```python
from build123d import *

# Parameters (mm, degrees)
PAD_DEPTH       = 5
CHAMFER_SIZE    = 3
SKETCH001_R     = 1.65
POCKET_DEPTH    = 5
FILLET_R        = 4
SKETCH002_R     = 1.7
POCKET001_DEPTH = 10.001
CHAMFER001_SIZE = 1.5


with BuildPart() as part:
    # Sketch → Pad (new body, symmetric)
    with BuildSketch(Plane.XY):
        Polygon((-27.5, 0), (0, 0), (0, 30), (-9, 30), (-9, 4), (-27.5, 4), align=None)
    extrude(amount=PAD_DEPTH, both=True)

    # Chamfer
    chamfer_edges = [part.edges().sort_by_distance(p)[0] for p in [
        (0, 0, 0),
    ]]
    chamfer(chamfer_edges, length=CHAMFER_SIZE)

    # Sketch001 (on Face7 of Chamfer) → Pocket (cut)
    with BuildSketch(Plane(origin=(0, 4, 0), x_dir=(-1, 0, 0), z_dir=(0, 1, 0))):
        with Locations((22.75, 0)):
            Circle(SKETCH001_R)
        with Locations((13.75, 0)):
            Circle(SKETCH001_R)
    extrude(amount=-POCKET_DEPTH, mode=Mode.SUBTRACT)

    # Fillet
    fillet_edges = [part.edges().sort_by_distance(p)[0] for p in [
        (-9, 30, 0),
        (0, 30, 0),
    ]]
    fillet(fillet_edges, radius=FILLET_R)

    # Sketch002 (on Face11 of Fillet) → Pocket001 (cut, through all)
    with BuildSketch(Plane.XY.offset(5)):
        with Locations((-4.5, 25)):
            Circle(SKETCH002_R)
    extrude(amount=-POCKET001_DEPTH, mode=Mode.SUBTRACT)

    # Chamfer001
    chamfer001_edges = [part.edges().sort_by_distance(p)[0] for p in [
        (-27.5, 4, 0),
    ]]
    chamfer(chamfer001_edges, length=CHAMFER001_SIZE)


solid = part.part
```
Geometry check sheet. Reference: the model listing, model coordinates, mm. A direction names the side the tool comes from. Give positions to 0.01 mm unless a question says otherwise; leave off trailing zeros. Order: outer loops, then holes, each group sorted by start corner. A loop starts at its lowest first (then second) coordinate and runs counter-clockwise, first axis right, second up.
1. Release check for a two-part mould opening along X. For faces 1 (the face through (-8, 12, -5)), 2 (the face through (-15.274, 2.028, -0.632)), 3 (the face through (-7.797, 28.859, 0.07)), 4 (the face through (-1, 2, 0)) record: pulls with the +X half, pulls with the -X half, needs draft (parallel to the pull), parting line crosses it, or undercut.
2. Section check B-B, the plane y = 25. Enter the section's corners in (x, z).
3. Access from +Z, -Z, +X, -X, +Y, -Y to the whole of each face (thin tool, end or side, straight path). Record for faces 5 (the face through (-15.4, 0, -1)), 6 (the face through (-9, 15, 0)).
4. Section check D-D, the plane z = 3.75. Enter the section's corners in (x, y).
5. Thickness scan on L1, parallel to Z at x = -22.75, y = 1.4; L2, parallel to Y at x = -4.5, z = 1.5; L3, parallel to X at y = 22.5, z = -1.75. Record the ranges inside material, lowest first.
6. Section check C-C, the plane x = -4.5. Enter the section's corners in (y, z), and give its area (3 significant figures).
7. Gauge pin test, flat ends, axial feed: pin 1 Ø5.5 at (x, z) = (-22.75, 0) entering from +Y; pin 2 Ø6 at (y, z) = (12.5, 2) entering from -X; pin 3 Ø3 at (x, y) = (-4.5, 25) entering from +Z. Record the tip position at first contact, or that the pin passes through.
8. Section check A-A, the plane z = 0. Enter the section's corners in (x, y), and give its area (3 significant figures).
Values follow:
1. face 1: needs draft
1. face 2: undercut
1. face 3: pulls with the -X half
1. face 4: pulls with the +X half
2. outline: (-9, -5) - (-6.2, -5) - (-6.2, 5) - (-9, 5) - close; (-2.8, -5) - (0, -5) - (0, 5) - (-2.8, 5) - close
3. face 5: +Z, -Z, +X, -X, -Y
3. face 6: +Z, -Z, -X, +Y
4. outline: (-27.5, 0) - (-3, 0) - (0, 3) - (0, 26) arc R4 ccw to (-4, 30) - (-5, 30) arc R4 ccw to (-9, 26) - (-9, 4) - (-26, 4) - (-27.5, 2.5) - close; hole circle Ø3.4 at (-4.5, 25)
5. L1: z = -5 to -1.65, 1.65 to 5
5. L2: y = 0 to 23.3, 26.7 to 30
5. L3: x = -9 to 0
6. outline: (0, -5) - (23.3, -5) - (23.3, 5) - (0, 5) - close; (26.7, -5) - (30, -5) - (30, 5) - (26.7, 5) - close
6. area: 266 mm2
7. pin 1: stops at y = 4
7. pin 2: stops at x = -9
7. pin 3: passes through
8. outline: (-27.5, 0) - (-24.4, 0) - (-24.4, 4) - (-26, 4) - (-27.5, 2.5) - close; (-21.1, 0) - (-15.4, 0) - (-15.4, 4) - (-21.1, 4) - close; (-12.1, 0) - (-3, 0) - (0, 3) - (0, 26) arc R4 ccw to (-4, 30) - (-5, 30) arc R4 ccw to (-9, 26) - (-9, 4) - (-12.1, 4) - close; hole circle Ø3.4 at (-4.5, 25)
8. area: 296 mm2
